from build123d import *

# Parameters (mm, degrees)
F0_W           = 100
F0_H           = 50
F0_R           = 17.029171721
F1_DEPTH       = 10
F3_DEPTH       = 20
F5_D           = 5
F5_DEPTH       = 12
F5_CSINK_D     = 10
F5_CSINK_ANGLE = 90
F5_TIP         = 1.5021515476
F7_D           = 5
F7_CSINK_D     = 10
F7_CSINK_ANGLE = 90
F8_T           = -2.5


with BuildPart() as f1:
    # F0 (on Front) → F1 (new body)
    with BuildSketch(Plane.XZ):
        with Locations((50, 25)):
            Rectangle(F0_W, F0_H)
        with Locations((26.453634724, 25)):
            Circle(F0_R, mode=Mode.SUBTRACT)
    extrude(amount=F1_DEPTH)

    # F2 (on face) → F3 (join)
    with BuildSketch(Plane.XZ.offset(10)):
        Polygon((93, 43), (53, 43), (53, 36), (83, 36), (83, 29), (68, 29), (68, 21), (83, 21), (83, 14), (53, 14), (53, 7), (93, 7), align=None)
    extrude(amount=F3_DEPTH)

    # F5
    with Locations(Plane(origin=(0, 0, 7), x_dir=(1, 0, 0), z_dir=(0, 0, -1))):
        with Locations((63, 20)):
            CounterSinkHole(F5_D / 2, F5_CSINK_D / 2, depth=F5_DEPTH, counter_sink_angle=F5_CSINK_ANGLE)
            with Locations((0, 0, -(F5_DEPTH + F5_TIP / 2))):  # 118° drill point
                Cone(0, F5_D / 2, F5_TIP, mode=Mode.SUBTRACT)

    # F7 (through all)
    with Locations(Plane.XY.offset(43)):
        with Locations((63, -20)):
            CounterSinkHole(F7_D / 2, F7_CSINK_D / 2, counter_sink_angle=F7_CSINK_ANGLE)

    # F8
    f8_openings = [f1.faces().sort_by_distance(p)[0] for p in [
        (55.246236, 0, 25),
    ]]
    offset(amount=F8_T, openings=f8_openings, kind=Kind.INTERSECTION)


solid = f1.part
Build history of the part. All positions in model axes, mm. A direction names the side the tool comes from. Coordinates: 2 decimals unless noted, no trailing zeros. Order: outer loops, then holes, each group sorted by start corner. A loop starts at its lowest first (then second) coordinate and runs counter-clockwise, first axis right, second up. Notation, with made-up numbers: (55.5, -4) -> (77.5, -4) arc R28 cw to (77.5, 22) -> close; hole circle Ø3 at (-18, 69.5). An arc over 180 degrees is marked (long way). One line per item, written item: value.
(1) Slice it at D-D, the plane x = 35.5. List the corners of the cut face in (y, z).
Checked values:
outline: (-10, 0) -> (0, 0) -> (0, 2.5) -> (-7.5, 2.5) -> (-7.5, 7.69) -> (0, 7.69) -> (0, 10.57) -> (-10, 10.57) -> close; (-10, 39.43) -> (0, 39.43) -> (0, 42.31) -> (-7.5, 42.31) -> (-7.5, 47.5) -> (0, 47.5) -> (0, 50) -> (-10, 50) -> close
(2) Tool access for faces 4 (the cylindrical face through (12.06, -3.7, 38.2)), 5 (the flat face through (76, -20, 29)), 6 (the flat face through (53, -20, 40)): list every direction of +Z, -Z, +X, -X, +Y, -Y with a clear straight run to the whole face (end or side of a thin tool).
Checked values:
face 4: +Y
face 5: -X, -Y
face 6: +Z, -Z, -X, -Y
(3) Slice it at A-A, the plane z = 25. List the corners of the cut face in (x, y).
Checked values:
outline: (0, -10) -> (9.42, -10) -> (9.42, 0) -> (6.92, 0) -> (6.92, -7.5) -> (2.5, -7.5) -> (2.5, 0) -> (0, 0) -> close; (43.48, -10) -> (68, -10) -> (68, -30) -> (93, -30) -> (93, -10) -> (100, -10) -> (100, 0) -> (97.5, 0) -> (97.5, -7.5) -> (90.5, -7.5) -> (90.5, -27.5) -> (70.5, -27.5) -> (70.5, -7.5) -> (45.98, -7.5) -> (45.98, 0) -> (43.48, 0) -> close
(4) Mould opens along Z. For faces 1 (the flat face through (49, -5, 50)), 2 (the flat face through (93, -20, 25)), 3 (the cylindrical face through (12.94, -4.93, 14.64)) say: pulls with the +Z half, pulls with the -Z half, needs draft (parallel to the pull), parting line crosses it, or undercut.
Checked values:
face 1: pulls with the +Z half
face 2: needs draft
face 3: undercut
(5) Probe line 1 (Z direction, x = 83.5, y = -20.25); line 2 (Z direction, x = 78.5, y = -22); line 3 (X direction, y = -20, z = 37.6). List the from-to ranges inside material, lowest first. Write a range as [from, to].
Checked values:
line 1: [7, 9.5], [11.5, 23.5], [26.5, 38.5], [40.5, 43]
line 2: [7, 9.5], [11.5, 14], [21, 23.5], [26.5, 29], [36, 38.5], [40.5, 43]
line 3: [53, 60.5], [65.5, 85.5], [90.5, 93]
(6) Drop flat-ended pins along their axis: pin 1 Ø9.5 at (y, z) = (-22.5, 18) entering from +X; pin 2 Ø5.5 at (y, z) = (-21, 33) entering from -X; pin 3 Ø4 at (x, y) = (63, -20) entering from +Z; pin 4 Ø16 at (x, y) = (79, -18.5) entering from +Z. Give the stop position or say it passes through.
Checked values:
pin 1: x = 93
pin 2: x = 83
pin 3: through
pin 4: z = 43
(7) Slice it at B-B, the plane y = -20. Count the separate pieces of the cut face and the enclosed holes in it, plus the area to 3 significant figures.
Checked values:
separate pieces: 3
enclosed holes: 3
area: 540 mm2
